Build history of the part. All positions in model axes, mm. A direction names the side the tool comes from. Round coordinates to 2 decimals unless told otherwise and drop trailing zeros. Loops run counter-clockwise (first coordinate to the right, second up) from the corner with the lowest first, then second, coordinate; pieces in that order, holes last. Notation, with made-up numbers: (-28, -8.75) -> (-2, -8.75) arc R13 cw to (-2, -4.75) -> close; hole circle Ø1 at (86, -17). An arc over 180 degrees is marked (long way). Put each result on its own line as item: value. Start each with the question number.
Item 1: Drill centre lines: probe 1 along Y at (x, z) = (-224.5, -12); probe 2 along Y at (x, z) = (-62.5, -150); probe 3 along Z at (x, y) = (19, -51.5). Where is each one in solid material? Low to high. Write a range as [from, to].
Item 2: Cut at D-D, the plane z = 338. List the corners of the cut face in (x, y).
Item 3: Pull direction X, two halves, no side cores. Call faces 3 (the flat face through (-20, -75, -164)), 4 (the flat face through (-89.11, -24.65, -18.48)), 5 (the flat face through (-232.338, -24.65, 302.162)): +X half, -X half, draft (parallel to the pull), parting line (faces both ways), or undercut.
Item 4: Cut at B-B, the plane x = 22. List the corners of the cut face in (y, z), plus the area to 3 significant figures.
Item 5: Cut at C-C, the plane z = -147. List the corners of the cut face in (x, y).
Item 6: Cut at A-A, the plane y = -23.5. List the corners of the cut face in (x, z).
Item 7: Tool access for faces 1 (the cylindrical face through (82.337, -62.325, -74.98)), 2 (the flat face through (-167.46, -24.65, 298.77)): list every direction of +Z, -Z, +X, -X, +Y, -Y with a clear straight run to the whole face (end or side of a thin tool).
Item 8: Flat gauge pins, fed straight in: pin 1 Ø1 at (x, y) = (-113, -21.5) entering from -Z; pin 2 Ø2 at (y, z) = (-32.5, -86) entering from +X; pin 3 Ø4 at (x, y) = (-151, -39) entering from -Z. Where does each tip first touch, or does it go through?
```python
from build123d import *

# Parameters (mm, degrees)
F1_DEPTH = 50
F2_R     = 86.3227416046
F3_DEPTH = 25
F4_R     = 65.7159407402
F5_DEPTH = 10


with BuildPart() as f1:
    # F0 (on Front) → F1 (new body)
    with BuildSketch(Plane.XZ):
        with BuildLine():
            ThreePointArc((-20.4931345241, -198.7868681146), (63.0503233441, -178.5278953222), (100, -100.9092330933))
            ThreePointArc((100, -100.9092330933), (68.9263499461, -28.4581579936), (-4.983165662, -1.0334699673))
            Line((-4.983165662, -1.0334699673), (-35.1463871142, -7.2890885045))
            ThreePointArc((-35.1463871142, -7.2890885045), (-99.7085201522, -108.5388470457), (-20.4931345241, -198.7868681146))
        make_face()
        with BuildLine():
            Line((-35.1463871142, -7.2890885045), (-4.983165662, -1.0334699673))
            ThreePointArc((-4.983165662, -1.0334699673), (-20.307103248, -2.9928322317), (-35.1463871142, -7.2890885045))
        make_face()
        with BuildLine():
            Line((-201.4895329203, -160.8907410076), (-20.4931345241, -198.7868681146))
            ThreePointArc((-20.4931345241, -198.7868681146), (-99.7085201522, -108.5388470457), (-35.1463871142, -7.2890885045))
            Line((-35.1463871142, -7.2890885045), (-144.6050883957, -29.989975473))
            Line((-144.6050883957, -29.989975473), (-140.1335041643, -96.908898563))
            ThreePointArc((-140.1335041643, -96.908898563), (-140.0333853292, -98.9079522711), (-140, -100.9092330933))
            ThreePointArc((-140, -100.9092330933), (-158.1035322206, -143.8590408648), (-201.4895329203, -160.8907410076))
        make_face()
        with BuildLine():
            ThreePointArc((-259.9795126124, -102.4770553995), (-242.3987093701, -143.3633193954), (-201.4895329203, -160.8907410076))
            ThreePointArc((-201.4895329203, -160.8907410076), (-158.1035322206, -143.8590408648), (-140, -100.9092330933))
            ThreePointArc((-140, -100.9092330933), (-140.0333853292, -98.9079522711), (-140.1335041643, -96.908898563))
            ThreePointArc((-140.1335041643, -96.908898563), (-158.1101162428, -57.9530037568), (-197.505495076, -40.9611101436))
            ThreePointArc((-197.505495076, -40.9611101436), (-237.9912102248, -54.4692939713), (-259.2537512084, -91.4756246778))
            Line((-259.2537512084, -91.4756246778), (-259.9795126124, -102.4770553995))
        make_face()
        with BuildLine():
            Line((-140.1335041643, -96.908898563), (-144.6050883957, -29.989975473))
            Line((-144.6050883957, -29.989975473), (-197.505495076, -40.9611101436))
            ThreePointArc((-197.505495076, -40.9611101436), (-158.1101162428, -57.9530037568), (-140.1335041643, -96.908898563))
        make_face()
        with BuildLine():
            Line((-197.505495076, -40.9611101436), (-144.6050883957, -29.989975473))
            Line((-144.6050883957, -29.989975473), (-160.0662830286, 201.3925594364))
            ThreePointArc((-160.0662830286, 201.3925594364), (-160.016574191, 200.2421402486), (-160, 199.0907669067))
            ThreePointArc((-160, 199.0907669067), (-201.1288321578, 159.1066983549), (-239.936286898, 201.3475320257))
            Line((-239.936286898, 201.3475320257), (-259.2537512084, -91.4756246778))
            ThreePointArc((-259.2537512084, -91.4756246778), (-237.9912102248, -54.4692939713), (-197.505495076, -40.9611101436))
        make_face()
        with BuildLine():
            ThreePointArc((-259.2537512084, -91.4756246778), (-259.8698644546, -96.9596343563), (-259.9795126124, -102.4770553995))
            Line((-259.9795126124, -102.4770553995), (-259.2537512084, -91.4756246778))
        make_face()
        with BuildLine():
            Line((-160.1150603833, 202.1225307119), (-160.0662830286, 201.3925594364))
            ThreePointArc((-160.0662830286, 201.3925594364), (-160.0890027762, 201.7576565936), (-160.1150603833, 202.1225307119))
        make_face()
        with BuildLine():
            ThreePointArc((-160, 199.0907669067), (-160.016574191, 200.2421402486), (-160.0662830286, 201.3925594364))
            Line((-160.0662830286, 201.3925594364), (-160.1150603833, 202.1225307119))
            ThreePointArc((-160.1150603833, 202.1225307119), (-200.0113479884, 239.090765297), (-239.8866534174, 202.0998995332))
            Line((-239.8866534174, 202.0998995332), (-239.936286898, 201.3475320257))
            ThreePointArc((-239.936286898, 201.3475320257), (-201.1288321578, 159.1066983549), (-160, 199.0907669067))
        make_face()
        with BuildLine():
            ThreePointArc((-239.8866534174, 202.0998995332), (-200.0113479884, 239.090765297), (-160.1150603833, 202.1225307119))
            Line((-160.1150603833, 202.1225307119), (-175.0170289676, 398.1681844469))
            ThreePointArc((-175.0170289676, 398.1681844469), (-200.6469460036, 374.0991390912), (-224.9972436015, 399.4619977333))
            Line((-224.9972436015, 399.4619977333), (-239.8866534174, 202.0998995332))
        make_face()
        with BuildLine():
            ThreePointArc((-239.8866534174, 202.0998995332), (-239.9132429698, 201.7238327314), (-239.936286898, 201.3475320257))
            Line((-239.936286898, 201.3475320257), (-239.8866534174, 202.0998995332))
        make_face()
        with BuildLine():
            ThreePointArc((-224.9972436015, 399.4619977333), (-200.6469460036, 374.0991390912), (-175.0170289676, 398.1681844469))
            ThreePointArc((-175.0170289676, 398.1681844469), (-175.0042576044, 398.6293971036), (-175, 399.0907669067))
            ThreePointArc((-175, 399.0907669067), (-198.3044384925, 424.033202056), (-224.7700056939, 402.4740815422))
            Line((-224.7700056939, 402.4740815422), (-224.9972436015, 399.4619977333))
        make_face()
        with BuildLine():
            ThreePointArc((-224.7700056939, 402.4740815422), (-224.9291583858, 400.9714747983), (-224.9972436015, 399.4619977333))
            Line((-224.9972436015, 399.4619977333), (-224.7700056939, 402.4740815422))
        make_face()
    extrude(amount=F1_DEPTH)

    # F2 (on face) → F3 (join)
    with BuildSketch(Plane.XZ.offset(50)):
        with Locations((0, -100.9092330933)):
            Circle(F2_R)
    extrude(amount=F3_DEPTH)

    # F4 (on face) → F5 (join)
    with BuildSketch(Plane.XZ.offset(75)):
        with Locations((0, -100.9092330933)):
            Circle(F4_R)
    extrude(amount=F5_DEPTH)


solid = f1.part
```
Reply:
1. probe 1: y = [-50, 0]
1. probe 2: y = [-75, 0]
1. probe 3: z = [-185.12, -16.7]
2. outline: (-229.63, -50) -> (-170.44, -50) -> (-170.44, 0) -> (-229.63, 0) -> close
3. face 3: draft
3. face 4: undercut
3. face 5: -X half
4. outline: (-85, -162.83) -> (-75, -162.83) -> (-75, -184.38) -> (-50, -184.38) -> (-50, -198.46) -> (0, -198.46) -> (0, -3.36) -> (-50, -3.36) -> (-50, -17.44) -> (-75, -17.44) -> (-75, -38.99) -> (-85, -38.99) -> close
4. area: 15,200 mm^2
5. outline: (-238.41, -50) -> (-72.99, -50) -> (-72.99, -75) -> (-46.84, -75) -> (-46.84, -85) -> (46.84, -85) -> (46.84, -75) -> (72.99, -75) -> (72.99, -50) -> (88.74, -50) -> (88.74, 0) -> (-238.41, 0) -> close
6. outline: (-259.25, -91.48) arc R60 ccw to (-201.49, -160.89) -> (-20.49, -198.79) arc R100 ccw (long way) to (-35.15, -7.29) -> (-144.61, -29.99) -> (-160.07, 201.39) arc R40 ccw to (-160.12, 202.12) -> (-175.02, 398.17) arc R25 ccw (long way) to (-225, 399.46) -> (-239.89, 202.1) arc R40 ccw to (-239.94, 201.35) -> close
7. face 1: -Y
7. face 2: +Z, +X, +Y, -Y
8. pin 1: stops at z = -179.52
8. pin 2: stops at x = 99.03
8. pin 3: stops at z = -171.88
